from build123d import *

# Parameters (mm, degrees)
F0_R     = 36.5
F0_W     = 4
F0_H     = 10
F1_DEPTH = 4
F0_R_2   = 40.5
F2_DEPTH = 55
F3_R     = 1.99999
F4_R     = 4


# Not quite as in the source:
# - a fillet or chamfer is up to 0.001 mm smaller than in the source, because OpenCascade refuses the exact size


with BuildPart() as f1:
    # F0 (on Top) → F1 (new body)
    with BuildSketch(Plane.XY):
        Circle(F0_R)
        with Locations((-27.25, -15.4073267064)):
            Rectangle(F0_W, F0_H, mode=Mode.SUBTRACT)
        with Locations((27.25, -14.5926732936)):
            Rectangle(F0_W, F0_H, mode=Mode.SUBTRACT)
        with Locations((-27.25, 14.5926732936)):
            Rectangle(F0_W, F0_H, mode=Mode.SUBTRACT)
        with Locations((27.25, 15.4073267064)):
            Rectangle(F0_W, F0_H, mode=Mode.SUBTRACT)
    extrude(amount=F1_DEPTH)

    # F0 (on Top) → F2 (join)
    with BuildSketch(Plane.XY):
        Circle(F0_R_2)
        Circle(F0_R, mode=Mode.SUBTRACT)
    extrude(amount=F2_DEPTH)

    # F3 (radius 2 in the source; OpenCascade refuses exactly that, so slightly less here)
    f3_edges = [f1.edges().sort_by_distance(p)[0] for p in [
        (-40.5, 0, 55),
        (-36.5, 0, 55),
    ]]
    fillet(f3_edges, radius=F3_R)

    # F4
    f4_edges = [f1.edges().sort_by_distance(p)[0] for p in [
        (-40.5, 0, 0),
    ]]
    fillet(f4_edges, radius=F4_R)


solid = f1.part
Verification items for the finished model (mm, model axes). A direction names the side the tool comes from. Coordinates: 2 decimals unless noted, no trailing zeros. Loops run counter-clockwise (first coordinate to the right, second up) from the corner with the lowest first, then second, coordinate; pieces in that order, holes last. Notation, with made-up numbers: (-5, 53) -> (11, 53) arc R7 ccw to (11, 66) -> close; hole circle Ø9 at (28.25, 39.5). An arc over 180 degrees is marked (long way). Answer as a JSON object with one key per item and string values. Group by question number.
Item 1: Depth check by flat-ended pin: pin 1 (3 mm diameter, centred on x = -28, z = 1, fed in from -Y); pin 2 (4 mm diameter, centred on y = 25, z = 13, fed in from +X); pin 3 (3 mm diameter, centred on x = 26.5, z = 1.5, fed in from -Y). Enter the tip coordinate at first touch or a pass-through.
Item 2: Sectioned sample at B-B on z = 5.5. Record the boundary of the cut face in (x, y), plus the area to 3 significant figures.
Item 3: Scan lines: probe 1 along Y at (x, z) = (0, 36); probe 2 along X at (y, z) = (13.5, 13); probe 3 along Z at (x, y) = (-1.5, -15). Record each from-to range of solid material in increasing order.
Item 4: Mould release check, pull along X, two halves, no side actions. Record for faces 3 (the cylindrical face through (21.77, 34.15, 28.16)), 4 (the flat face through (-27, -10.407, 2)): +X half, -X half, draft (parallel to the pull), parting line (faces both ways), or undercut.
Item 5: Sectioned sample at D-D on y = -17. State how many separate pieces and enclosed holes the cut face has, plus the area to 3 significant figures.
Item 6: Tool access check on faces 1 (the cylindrical face through (-7.912, -35.632, 28.157)), 2 (the flat face through (29.25, -15, 2)). Record the directions out of +Z, -Z, +X, -X, +Y, -Y that give a thin tool (end or side, any length) a straight path to the whole face; none if there is none.
Evaluation:
{
 "1": {"pin 1": "stops at y = -29.57", "pin 2": "stops at x = 33.34", "pin 3": "stops at y = -31.2"},
 "2": {"outline": "circle Ø81 at (0, 0); hole circle Ø73 at (0, 0)", "area": "968 mm²"},
 "3": {"probe 1": "y = -40.5 to -36.5, 36.5 to 40.5", "probe 2": "x = -38.18 to -33.91, 33.91 to 38.18", "probe 3": "z = 0 to 4"},
 "4": {"face 3": "parting line", "face 4": "undercut"},
 "5": {"separate pieces": "3", "enclosed holes": "0", "area": "706 mm²"},
 "6": {"face 1": "+Z", "face 2": "+Z, -Z"}
}
